The listing builds one solid part. Answer for the finished solid, in the listing's coordinates (mm). A direction names the side the tool comes from. Round coordinates to 2 decimals unless told otherwise and drop trailing zeros. Order: outer loops, then holes, each group sorted by start corner. A loop starts at its lowest first (then second) coordinate and runs counter-clockwise, first axis right, second up. Notation, with made-up numbers: (-18.75, -28) - (-13.75, -28) arc R30 ccw to (-13.75, 10) - close; hole circle Ø11 at (77.5, -13). An arc over 180 degrees is marked (long way). One line per item, written item: value. Start each with the question number.
1. Section B-B, the plane x = 381 is taken. Give the vertices of the cut face in (y, z).
2. Flat-ended cylindrical pins translate along their axes: P1, Ø3.5, axis at x = 299.65, z = 97.24, coming from the +Y side; P2, Ø4, axis at x = 448, z = 125.5, coming from the -Y side; P3, Ø6, axis at x = 257.5, z = 115.5, coming from the +Y side. Find the tip coordinate at first contact, or state that the pin passes through.
3. Section C-C, the plane z = 53.5 is taken. Give the vertices of the cut face in (x, y), then the cut area to 3 significant figures.
4. A tool of negligible diameter and unlimited length cuts with its end or side. For faces 1 (the flat face through (387.128, 0.715, 45.424)), 2 (the flat face through (341.894, 3.605, -54.278)), 3 (the flat face through (390.9, 0.17, 18.64)), 4 (the flat face through (318.666, -1.521, -14.045)), 5 (the flat face through (415.9, 0.17, 61.94)), from which of +Z, -Z, +X, -X, +Y, -Y can it reach the whole face along a straight path? Write none if from no direction.
5. Straight lines are drawn through the part: line 1 (Z direction, x = 352, y = 2.5); line 2 (Y direction, x = 309.5, z = 21.5); line 3 (Z direction, x = 294, y = -0.75). For each, find the intervals that lie inside material, in ascending order.
6. For a pull along X with two mould halves and no side action, classify faces 6 (the flat face through (301, 1, 46)), 7 (the flat face through (304.924, 0.168, 16.426)), 8 (the flat face through (388.8, -3.49, 48.32)), 9 (the flat face through (447, 11, 127)) as released by +X, released by -X, zero draft, split by the parting line, or undercut.
7. Section A-A, the plane y = 8.75 is taken. Give the vertices of the cut face in (x, z), then the cut area to 3 significant figures.
8. Section D-D, the plane z = -51 is taken. Give the vertices of the cut face in (x, y), then the cut area to 3 significant figures.
from build123d import *

# Parameters (mm, degrees)
SKETCH1_W                = 34.714871787
SKETCH1_H                = 10.923666426
BOSS_EXTRUDE1_DEPTH      = 1
BOSS_EXTRUDE2_DEPTH      = 11
BOSS_EXTRUDE3_DEPTH      = 5
BOSS_EXTRUDE3_DEPTH_BACK = 3
SKETCH3_W                = 50
SKETCH3_H                = 7
CUT_EXTRUDE3_DEPTH       = 25
SKETCH5_W                = 50
SKETCH5_H                = 7
CUT_EXTRUDE4_DEPTH       = 25
SKETCH6_W                = 50
SKETCH6_H                = 7
CUT_EXTRUDE5_DEPTH       = 25
SKETCH8_R                = 1.5
BOSS_EXTRUDE5_DEPTH      = 1
BOSS_EXTRUDE10_DEPTH     = 3


with BuildPart() as part:
    # Sketch1 → Boss-Extrude1 (new body)
    with BuildSketch(Plane(origin=(0, 0, 0), x_dir=(1, 0, 0), z_dir=(0, 1, 0))):
        Polygon((243.304219775, -116.484791865), (254.809280577, -136.408896137), (442.602090749, -136.409305398), (444.621046679, -132.925433224), (441.749040748, -132.925433224), (449.516726724, -119.471406458), (450.964695298, -121.978953123), (452.699916622, -118.984688018), (358.778179036, 43.666038065), (335.767496284, 43.666038065), align=None)
        with Locations((422.370878913, -129.522754792)):
            Rectangle(SKETCH1_W, SKETCH1_H, mode=Mode.SUBTRACT)
        Polygon((423.190377512, -92.577472767), (432.651287025, -87.114324326), (450.119365975, -117.364996826), (440.658456462, -122.828145267), align=None, mode=Mode.SUBTRACT)
        Polygon((428.113670919, -116.417164681), (266.439108268, -116.428009237), (347.273609729, 23.609230821), align=None, mode=Mode.SUBTRACT)
    extrude(amount=BOSS_EXTRUDE1_DEPTH)

    # Sketch1_9 → Boss-Extrude2 (add)
    # profile 1 of 2: a face of its own
    with BuildSketch(Plane(origin=(0, 0, 0), x_dir=(1, 0, 0), z_dir=(0, 1, 0))):
        Polygon((229.159432548, -134.984249184), (231.716666588, -139.412373829), (462.829865412, -139.412373829), (465.38624875, -134.984588004), (349.829542096, 65.165499075), (344.716133219, 65.165499075), align=None)
        Polygon((251.922647989, -136.409305399), (233.446303401, -136.408896138), (232.62355396, -134.984217357), (241.860901689, -118.984688018), align=None, mode=Mode.SUBTRACT)
        Polygon((442.602090749, -136.409305398), (254.809280577, -136.408896137), (243.304219775, -116.484791865), (335.767496284, 43.666038065), (358.778179036, 43.666038065), (461.938967958, -134.984588006), (461.116393749, -136.409305398), align=None, mode=Mode.SUBTRACT)
        Polygon((348.096628302, 62.164013367), (357.334800991, 46.166038067), (337.210874326, 46.166038067), (346.44844193, 62.165948237), align=None, mode=Mode.SUBTRACT)
    # profile 2 of 2: a face of its own
    with BuildSketch(Plane(origin=(0, 0, 0), x_dir=(1, 0, 0), z_dir=(0, 1, 0))):
        Polygon((441.749040748, -132.925433224), (444.621046679, -132.925433224), (450.964695298, -121.978953123), (449.516726724, -119.471406458), align=None)
    extrude(amount=BOSS_EXTRUDE2_DEPTH)

    # Sketch1_10 → Boss-Extrude3 (add, two sides: drawn at the far end of the back side and taken through both)
    # profile 1 of 2: a face of its own
    with BuildSketch(Plane(origin=(0, 0, 0), x_dir=(1, 0, 0), z_dir=(0, 1, 0)).offset(-BOSS_EXTRUDE3_DEPTH_BACK)):
        Polygon((229.159432548, -134.984249184), (231.716666588, -139.412373829), (462.829865412, -139.412373829), (465.38624875, -134.984588004), (349.829542096, 65.165499075), (344.716133219, 65.165499075), align=None)
        Polygon((251.922647989, -136.409305399), (233.446303401, -136.408896138), (232.62355396, -134.984217357), (241.860901689, -118.984688018), align=None, mode=Mode.SUBTRACT)
        Polygon((442.602090749, -136.409305398), (254.809280577, -136.408896137), (243.304219775, -116.484791865), (335.767496284, 43.666038065), (358.778179036, 43.666038065), (461.938967958, -134.984588006), (461.116393749, -136.409305398), align=None, mode=Mode.SUBTRACT)
        Polygon((348.096628302, 62.164013367), (357.334800991, 46.166038067), (337.210874326, 46.166038067), (346.44844193, 62.165948237), align=None, mode=Mode.SUBTRACT)
    # profile 2 of 2: a face of its own
    with BuildSketch(Plane(origin=(0, 0, 0), x_dir=(1, 0, 0), z_dir=(0, 1, 0)).offset(-BOSS_EXTRUDE3_DEPTH_BACK)):
        Polygon((441.749040748, -132.925433224), (444.621046679, -132.925433224), (450.964695298, -121.978953123), (449.516726724, -119.471406458), align=None)
    extrude(amount=BOSS_EXTRUDE3_DEPTH + BOSS_EXTRUDE3_DEPTH_BACK)

    # Sketch3 → Cut-Extrude3 (cut)
    with BuildSketch(Plane(origin=(290.589645397, 0, -167.772009994), x_dir=(-0.49999999999998745, 0, -0.8660254037844459), z_dir=(0.8660254037844459, 0, -0.49999999999998745))):
        with Locations((-236.592990632, -3)):
            Rectangle(SKETCH3_W, SKETCH3_H)
    extrude(amount=-CUT_EXTRUDE3_DEPTH, mode=Mode.SUBTRACT)

    # Sketch5 → Cut-Extrude4 (cut)
    with BuildSketch(Plane.XY.offset(139.412373829)):
        with Locations((347.273266, -3)):
            Rectangle(SKETCH5_W, SKETCH5_H)
    extrude(amount=-CUT_EXTRUDE4_DEPTH, mode=Mode.SUBTRACT)

    # Sketch6 → Cut-Extrude5 (cut)
    with BuildSketch(Plane(origin=(230.319375798, 0, 132.975171837), x_dir=(-0.5000006154012504, 0, 0.8660250484820695), z_dir=(-0.8660250484820695, 0, -0.5000006154012504))):
        with Locations((-113.236674799, -3)):
            Rectangle(SKETCH6_W, SKETCH6_H)
    extrude(amount=-CUT_EXTRUDE5_DEPTH, mode=Mode.SUBTRACT)

    # Sketch8 → Boss-Extrude5 (add)
    with BuildSketch(Plane.XZ.offset(3)):
        Polygon((349.829542096, -65.165499075), (465.38624875, 134.984588004), (462.829865412, 139.412373829), (231.716666588, 139.412373829), (229.159432548, 134.984249184), (344.716133219, -65.165499075), align=None)
        with Locations(Location((395.323540807, 98.692824234, 0), (0, 0, 270))):
            Circle(SKETCH8_R, mode=Mode.SUBTRACT)
        with Locations(Location((348.301285091, 15.863526629, 0), (0, 0, 270))):
            Circle(SKETCH8_R, mode=Mode.SUBTRACT)
        with Locations(Location((299.654911442, 97.24168178, 0), (0, 0, 270))):
            Circle(SKETCH8_R, mode=Mode.SUBTRACT)
        Polygon((450.14703547, 123.280701064), (452.699916622, 118.984688018), (461.938967958, 134.984588006), (461.116393749, 136.409305398), (442.602090749, 136.409305398), (445.226665069, 131.986443715), (401.697951811, 107.384591709), (406.618322213, 98.678849058), align=None, mode=Mode.SUBTRACT)
        Polygon((322.273266, 116.42426408), (294.358218631, 68.061097964), (319.354499367, 24.757680453), (376.473657316, 26.969372806), (401.47267951, 70.271207531), (372.273266, 116.420910257), align=None, mode=Mode.SUBTRACT)
        Polygon((233.446303401, 136.408896138), (251.922647989, 136.409305399), (241.860901689, 118.984688018), (232.62355396, 134.984217357), align=None, mode=Mode.SUBTRACT)
        Polygon((337.210874326, -46.166038067), (357.334800991, -46.166038067), (348.096628302, -62.164013367), (346.44844193, -62.165948237), align=None, mode=Mode.SUBTRACT)
    extrude(amount=BOSS_EXTRUDE5_DEPTH)

    # Sketch12 → Boss-Extrude10 (add)
    with BuildSketch(Plane(origin=(0, -3, 0), x_dir=(1, 0, 0), z_dir=(0, 1, 0))):
        with BuildLine():
            Line((347.417900211, -11.962292061), (347.307477101, -11.47463774))
            ThreePointArc((347.307477101, -11.47463774), (345.119304576, -12.681546114), (343.912396202, -14.869718639))
            Line((343.912396203, -14.869718639), (344.400050524, -14.980141749))
            ThreePointArc((344.400050523, -14.980141749), (345.472857967, -13.035099504), (347.417900211, -11.962292061))
        make_face()
        with BuildLine():
            ThreePointArc((352.690173981, -14.869718639), (351.483265607, -12.681546114), (349.295093082, -11.47463774))
            Line((349.295093081, -11.47463774), (349.184669971, -11.962292061))
            ThreePointArc((349.184669972, -11.962292061), (351.129712216, -13.035099504), (352.20251966, -14.980141749))
            Line((352.202519659, -14.980141749), (352.69017398, -14.869718639))
        make_face()
        with BuildLine():
            ThreePointArc((349.295093082, -20.252415518), (351.483265607, -19.045507145), (352.690173981, -16.857334619))
            Line((352.69017398, -16.857334619), (352.202519659, -16.746911509))
            ThreePointArc((352.20251966, -16.746911509), (351.129712216, -18.691953754), (349.184669972, -19.764761197))
            Line((349.184669971, -19.764761197), (349.295093081, -20.252415518))
        make_face()
        with BuildLine():
            Line((344.400050524, -16.746911509), (343.912396203, -16.857334619))
            ThreePointArc((343.912396202, -16.857334619), (345.119304576, -19.045507145), (347.307477101, -20.252415518))
            Line((347.307477101, -20.252415518), (347.417900211, -19.764761197))
            ThreePointArc((347.417900211, -19.764761197), (345.472857967, -18.691953754), (344.400050523, -16.746911509))
        make_face()
        with BuildLine():
            Line((394.440155927, -94.791589666), (394.329732817, -94.303935345))
            ThreePointArc((394.329732817, -94.303935345), (392.141560292, -95.510843718), (390.934651918, -97.699016244))
            Line((390.934651918, -97.699016244), (391.4247896, -97.798542945))
            ThreePointArc((391.4247896, -97.798542945), (392.499067689, -95.860448622), (394.440155927, -94.791589666))
        make_face()
        with BuildLine():
            ThreePointArc((399.712429696, -97.699016244), (398.505521323, -95.510843718), (396.317348797, -94.303935345))
            Line((396.317348797, -94.303935345), (396.206925687, -94.791589666))
            ThreePointArc((396.206925687, -94.791589666), (398.151967932, -95.864397109), (399.224775375, -97.809439354))
            Line((399.224775375, -97.809439354), (399.712429696, -97.699016244))
        make_face()
        with BuildLine():
            ThreePointArc((396.317348797, -103.081713123), (398.505521323, -101.874804749), (399.712429696, -99.686632224))
            Line((399.712429696, -99.686632224), (399.224775375, -99.576209114))
            ThreePointArc((399.224775375, -99.576209114), (398.151967932, -101.521251358), (396.206925687, -102.594058802))
            Line((396.206925687, -102.594058801), (396.317348797, -103.081713122))
        make_face()
        with BuildLine():
            Line((391.422306239, -99.576209114), (390.934651918, -99.686632224))
            ThreePointArc((390.934651918, -99.686632224), (392.141560292, -101.874804749), (394.329732817, -103.081713123))
            Line((394.329732817, -103.081713122), (394.440155927, -102.594058801))
            ThreePointArc((394.440155927, -102.594058802), (392.495113682, -101.521251358), (391.422306239, -99.576209114))
        make_face()
        with BuildLine():
            ThreePointArc((298.661103452, -92.852792892), (296.472930927, -94.059701265), (295.266022553, -96.24787379))
            Line((295.266022553, -96.24787379), (295.753676874, -96.3582969))
            ThreePointArc((295.753676874, -96.3582969), (296.826484317, -94.413254656), (298.771526562, -93.340447213))
            Line((298.771526562, -93.340447212), (298.661103452, -92.852792891))
        make_face()
        with BuildLine():
            ThreePointArc((304.04380033, -96.24787379), (302.836891957, -94.059701265), (300.648719432, -92.852792892))
            Line((300.648719432, -92.852792891), (300.538296322, -93.340447212))
            ThreePointArc((300.538296322, -93.340447213), (302.483338566, -94.413254656), (303.55614601, -96.3582969))
            Line((303.55614601, -96.3582969), (304.043800331, -96.24787379))
        make_face()
        with BuildLine():
            Line((300.538296322, -101.142916348), (300.648719432, -101.630570669))
            ThreePointArc((300.648719432, -101.630570669), (302.836891957, -100.423662295), (304.04380033, -98.23548977))
            Line((304.043800331, -98.23548977), (303.55614601, -98.12506666))
            ThreePointArc((303.55614601, -98.12506666), (302.483338566, -100.070108905), (300.538296322, -101.142916348))
        make_face()
        with BuildLine():
            Line((295.753676874, -98.12506666), (295.266022553, -98.23548977))
            ThreePointArc((295.266022553, -98.23548977), (296.472930927, -100.423662295), (298.661103452, -101.630570669))
            Line((298.661103452, -101.630570669), (298.771526562, -101.142916348))
            ThreePointArc((298.771526562, -101.142916348), (296.826484317, -100.070108905), (295.753676874, -98.12506666))
        make_face()
    extrude(amount=BOSS_EXTRUDE10_DEPTH)


solid = part.part
Answer list:
1. outline: (-4, -11.18) - (11, -11.18) - (11, -5.18) - (1, -5.18) - (1, 34.81) - (0.5, 34.81) - (0.5, 24.36) - (0, 24.36) - (0, -5.18) - (-3, -5.18) - (-3, 34.81) - (-4, 34.81) - close; (-4, 102.63) - (-3, 102.63) - (-3, 136.41) - (0, 136.41) - (0, 116.42) - (1, 116.42) - (1, 136.41) - (11, 136.41) - (11, 139.41) - (-4, 139.41) - close
2. P1: stops at y = -3
2. P2: stops at y = -3
2. P3: stops at y = 1
3. outline: (276.2, -4) - (302.76, -4) - (302.76, -3) - (276.2, -3) - close; (276.2, 0.5) - (302.76, 0.5) - (302.76, 1) - (279.67, 1) - (279.67, 11) - (276.2, 11) - close; (391.79, -4) - (418.34, -4) - (418.34, -3) - (391.79, -3) - close; (391.79, 0.5) - (418.34, 0.5) - (418.34, 11) - (414.89, 11) - (414.89, 1) - (391.79, 1) - close
3. area: 149 mm²
4. face 1: +Y
4. face 2: +Y, -Y
4. face 3: +X
4. face 4: none
4. face 5: -Z
5. line 1: z = -61.41 to -55.4, -46.17 to -43.67, 136.41 to 139.41
5. line 2: y = -4 to -3, 0.5 to 1
5. line 3: z = 136.41 to 139.41
6. face 6: undercut
6. face 7: released by -X
6. face 8: undercut
6. face 9: zero draft
7. outline: (229.16, 134.98) - (344.72, -65.17) - (349.83, -65.17) - (465.39, 134.98) - (462.83, 139.41) - (231.72, 139.41) - close; (441.75, 132.93) - (449.52, 119.47) - (450.96, 121.98) - (444.62, 132.93) - close; hole (232.62, 134.98) - (241.86, 118.98) - (251.92, 136.41) - (233.45, 136.41) - close; hole (243.3, 116.48) - (335.77, -43.67) - (358.78, -43.67) - (461.94, 134.98) - (461.12, 136.41) - (442.6, 136.41) - (254.81, 136.41) - close; hole (337.21, -46.17) - (346.45, -62.17) - (348.1, -62.16) - (357.33, -46.17) - close
7. area: 2,240 mm²
8. outline: (336.54, -4) - (340, -4) - (340, 11) - (336.54, 11) - close; (354.54, -4) - (358.01, -4) - (358.01, 11) - (354.54, 11) - close
8. area: 104 mm²
